Model file for the job. Use its own axes, mm. A direction names the side the tool comes from. Give positions to 0.01 mm unless a question says otherwise; leave off trailing zeros. Write each loop counter-clockwise with the first axis right and the second up, starting at its lowest first coordinate (ties: lowest second). Pieces come first, ordered by that corner, then holes. Notation, with made-up numbers: M 73.5,-8 L 97.5,-8 A37 ccw 97.5,30 Z; hole C 82,-29.5 d5. An arc over 180 degrees is marked long. Answer as a JSON object with one key per item and string values. Group by question number.
```python
from build123d import *

# Parameters (mm, degrees)
BOSS_EXTRUDE1_DEPTH  = 3
M3_CLEARANCE_HOLE1_D = 3.02
FILLET1_R            = 5


with BuildPart() as part:
    # Sketch1 → Boss-Extrude1 (new body)
    with BuildSketch(Plane(origin=(0, 0, 0), x_dir=(1, 0, 0), z_dir=(0, 1, 0))):
        Polygon((-17, 12), (17, 12), (17, 14), (25, 14), (25, 0), (-25, 0), (-25, 14), (-17, 14), align=None)
    extrude(amount=BOSS_EXTRUDE1_DEPTH)

    # M3 Clearance Hole1 (through all)
    with Locations(Plane(origin=(0, 3, 0), x_dir=(1, 0, 0), z_dir=(0, 1, 0))):
        with Locations((20, 5), (-20, 5)):
            Hole(M3_CLEARANCE_HOLE1_D / 2)

    # Fillet1
    fillet1_edges = [part.edges().sort_by_distance(p)[0] for p in [
        (25, 1.5, 0),
        (-25, 1.5, 0),
    ]]
    fillet(fillet1_edges, radius=FILLET1_R)


solid = part.part
```
Q1. Drop a flat-ended pin along its axis: P1, Ø1.5, axis at x = 7.5, y = 2, coming from the -Z side. Give the stop position or say it passes through.
Q2. 3-axis set-ups, long thin cutter, end or side, ignore diameter. For faces 1 (the flat face through (0, 3, -7)), 2 (the flat face through (-17, 1, -13)): which of +Z, -Z, +X, -X, +Y, -Y reach the whole face in a straight line?
Q3. Slice it at B-B, the plane y = 1.4. Write the cut outline in (x, z).
Q4. Slice it at C-C, the plane x = -19. Write the cut outline in (y, z), then the cut area to 3 significant figures.
Q5. Slice it at A-A, the plane z = -12.75. Write the cut outline in (x, y).
Q6. Wall check: L1, parallel to Z at x = -20, y = 2.35; L2, parallel to X at y = 2.3, z = -4.5; L3, parallel to X at y = 0.55, z = -4.75. Give the ranges that are in metal, low to high.
Q7. Two-plate mould, pull along Z, no slides. Class faces 3 (the flat face through (0, 1, 0)), 4 (the cylindrical face through (-20.812, 1.479, -6.273)), 5 (the flat face through (-25, 1, -9)): +Z half, -Z half, draft (parallel to the pull), parting line (faces both ways), or undercut.
Q8. Slice it at D-D, the plane z = -4.25. Write the cut outline in (x, y), then the cut area to 3 significant figures.
Solved:
{
 "1": {"P1": "stops at z = -12"},
 "2": {"face 1": "+Z, -Z, +X, -X, +Y", "face 2": "-Z, +Y, -Y"},
 "3": {"outline": "M -25,-14 L -17,-14 L -17,-12 L 17,-12 L 17,-14 L 25,-14 L 25,-5 A5 ccw 20,0 L -20,0 A5 ccw -25,-5 Z; hole C -20,-5 d3.02; hole C 20,-5 d3.02"},
 "4": {"outline": "M 0,-14 L 3,-14 L 3,-6.13 L 0,-6.13 Z; M 0,-3.87 L 3,-3.87 L 3,0 L 0,0 Z", "area": "35.2 mm²"},
 "5": {"outline": "M -25,0 L -17,0 L -17,3 L -25,3 Z; M 17,0 L 25,0 L 25,3 L 17,3 Z"},
 "6": {"L1": "z = -14 to -6.51, -3.49 to 0", "L2": "x = -24.97 to -21.42, -18.58 to 18.58, 21.42 to 24.97", "L3": "x = -24.99 to -21.49, -18.51 to 18.51, 21.49 to 24.99"},
 "7": {"face 3": "+Z half", "face 4": "undercut", "face 5": "draft"},
 "8": {"outline": "M -24.94,0 L -21.31,0 L -21.31,3 L -24.94,3 Z; M -18.69,0 L 18.69,0 L 18.69,3 L -18.69,3 Z; M 21.31,0 L 24.94,0 L 24.94,3 L 21.31,3 Z", "area": "134 mm²"}
}
